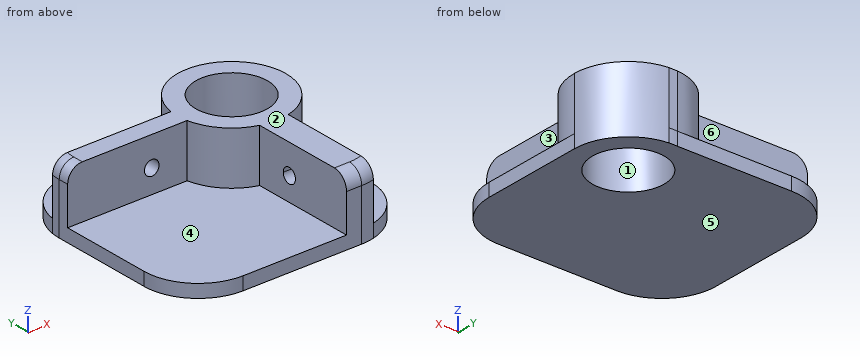
from build123d import *

# Parameters (mm, degrees)
F0_R     = 13.35
F1_DEPTH = 4.5
F2_DEPTH = 18
F5_DEPTH = 63.468562
F6_DEPTH = 56.501
F7_R     = 5
F8_R     = 13.35
F8_R_2   = 12.25
F9_DEPTH = 22.5


with BuildPart() as f1:
    # F0 (on Top) → F1 (new body)
    with BuildSketch(Plane.XY):
        with BuildLine():
            ThreePointArc((6.94, -57.959298), (17.066915, -51.404166), (21, -40))
            Line((21, -40), (21, -5))
            ThreePointArc((21, -5), (17.066915, -16.404166), (6.94, -22.959298))
            Line((6.94, -22.959298), (6.94, -57.959298))
        make_face()
        with Locations((2.5, -5)):
            Circle(F0_R)
        with BuildLine():
            ThreePointArc((6.94, -22.959298), (17.066915, -16.404166), (21, -5))
            ThreePointArc((21, -5), (16.086734, 7.555902), (3.956684, 13.442561))
            Line((3.956684, 13.442561), (1.066985, 13.444416))
            ThreePointArc((1.066985, 13.444416), (-10.011528, 8.627607), (-15.755136, -2))
            ThreePointArc((-15.755136, -2), (-15.998257, -5.25395), (-15.665902, -8.5))
            ThreePointArc((-15.665902, -8.5), (-11.178256, -17.456136), (-2.68, -22.76))
            ThreePointArc((-2.68, -22.76), (2.116816, -23.496031), (6.94, -22.959298))
        make_face()
        with Locations((2.5, -5)):
            Circle(F0_R, mode=Mode.SUBTRACT)
        with BuildLine():
            ThreePointArc((2.5, -58.5), (4.736401, -58.364327), (6.94, -57.959298))
            Line((6.94, -57.959298), (6.94, -22.959298))
            ThreePointArc((6.94, -22.959298), (2.116816, -23.496031), (-2.68, -22.76))
            Line((-2.68, -22.76), (-2.68, -58.5))
            Line((-2.68, -58.5), (2.5, -58.5))
        make_face()
        with BuildLine():
            Line((1.066985, 13.444416), (3.956684, 13.442561))
            ThreePointArc((3.956684, 13.442561), (2.511871, 13.499996), (1.066985, 13.444416))
        make_face()
        with BuildLine():
            ThreePointArc((-15.755136, -2), (-10.011528, 8.627607), (1.066985, 13.444416))
            Line((1.066985, 13.444416), (-38.015691, 13.469493))
            ThreePointArc((-38.015691, 13.469493), (-49.985176, 9.085639), (-56.277659, -2))
            Line((-56.277659, -2), (-15.755136, -2))
        make_face()
        with BuildLine():
            Line((-2.68, -58.5), (-2.68, -22.76))
            ThreePointArc((-2.68, -22.76), (-11.178256, -17.456136), (-15.665902, -8.5))
            Line((-15.665902, -8.5), (-56.527562, -8.5))
            Line((-56.527562, -8.5), (-56.527562, -40))
            ThreePointArc((-56.527562, -40), (-51.109037, -53.081475), (-38.027562, -58.5))
            Line((-38.027562, -58.5), (-2.68, -58.5))
        make_face()
        with BuildLine():
            ThreePointArc((-15.665902, -8.5), (-15.998257, -5.25395), (-15.755136, -2))
            Line((-15.755136, -2), (-56.277659, -2))
            ThreePointArc((-56.277659, -2), (-56.46498, -3.510108), (-56.527562, -5.030503))
            Line((-56.527562, -5.030503), (-56.527562, -8.5))
            Line((-56.527562, -8.5), (-15.665902, -8.5))
        make_face()
    extrude(amount=-F1_DEPTH)

    # F0 (on Top) → F2 (join)
    with BuildSketch(Plane.XY):
        with BuildLine():
            ThreePointArc((2.5, -58.5), (4.736401, -58.364327), (6.94, -57.959298))
            Line((6.94, -57.959298), (6.94, -22.959298))
            ThreePointArc((6.94, -22.959298), (2.116816, -23.496031), (-2.68, -22.76))
            Line((-2.68, -22.76), (-2.68, -58.5))
            Line((-2.68, -58.5), (2.5, -58.5))
        make_face()
        with BuildLine():
            ThreePointArc((6.94, -22.959298), (17.066915, -16.404166), (21, -5))
            ThreePointArc((21, -5), (16.086734, 7.555902), (3.956684, 13.442561))
            Line((3.956684, 13.442561), (1.066985, 13.444416))
            ThreePointArc((1.066985, 13.444416), (-10.011528, 8.627607), (-15.755136, -2))
            ThreePointArc((-15.755136, -2), (-15.998257, -5.25395), (-15.665902, -8.5))
            ThreePointArc((-15.665902, -8.5), (-11.178256, -17.456136), (-2.68, -22.76))
            ThreePointArc((-2.68, -22.76), (2.116816, -23.496031), (6.94, -22.959298))
        make_face()
        with Locations((2.5, -5)):
            Circle(F0_R, mode=Mode.SUBTRACT)
        with BuildLine():
            ThreePointArc((-15.665902, -8.5), (-15.998257, -5.25395), (-15.755136, -2))
            Line((-15.755136, -2), (-56.277659, -2))
            ThreePointArc((-56.277659, -2), (-56.46498, -3.510108), (-56.527562, -5.030503))
            Line((-56.527562, -5.030503), (-56.527562, -8.5))
            Line((-56.527562, -8.5), (-15.665902, -8.5))
        make_face()
    extrude(amount=F2_DEPTH)

    # F3 (on face) → F5 (cut, through all)
    with BuildSketch(Plane.YZ.offset(6.94)):
        with BuildLine():
            ThreePointArc((-32.459298, 8), (-33.191531, 9.767767), (-34.959298, 10.5))
            ThreePointArc((-34.959298, 10.5), (-36.727065, 6.232233), (-32.459298, 8))
        make_face()
    extrude(amount=-F5_DEPTH, mode=Mode.SUBTRACT)

    # F4 (on face) → F6 (cut, through all)
    with BuildSketch(Plane(origin=(0, -2, 0), x_dir=(-1, 0, 0), z_dir=(0, 1, 0))):
        with BuildLine():
            ThreePointArc((30.255136, 8), (29.522903, 9.767767), (27.755136, 10.5))
            ThreePointArc((27.755136, 10.5), (25.987369, 6.232233), (30.255136, 8))
        make_face()
    extrude(amount=-F6_DEPTH, mode=Mode.SUBTRACT)

    # F7
    f7_edges = [f1.edges().sort_by_distance(p)[0] for p in [
        (-56.527562, -6.765252, 18),
        (-0.09, -58.5, 18),
        (4.736401, -58.364327, 18),
    ]]
    fillet(f7_edges, radius=F7_R)

    # F8 (on face) → F9 (join, through all)
    with BuildSketch(Plane.XY.offset(18)):
        with Locations((2.5, -5)):
            Circle(F8_R)
        with Locations((2.5, -5)):
            Circle(F8_R_2, mode=Mode.SUBTRACT)
    extrude(amount=-F9_DEPTH)


solid = f1.part
The model under review builds one solid part; all positions refer to its coordinate system, in mm. Face numbers are marked on the shaded views. A direction names the side the tool comes from. Round coordinates to 2 decimals unless told otherwise and drop trailing zeros. Loops run counter-clockwise (first coordinate to the right, second up) from the corner with the lowest first, then second, coordinate; pieces in that order, holes last. Notation, with made-up numbers: M 49.5,45 L 76.5,45 A14 cw 76.5,51 Z; hole C 31,38 d11. An arc over 180 degrees is marked long. Answer as CSV lines item,"result". Start each with the question number.
Item 1: Wall thickness on line 1 (Y direction, x = 2.5, z = 1.75); line 2 (X direction, y = -6.75, z = 8); line 3 (Z direction, x = -28, y = -6): over which ranges is each line inside the solid? List them lowest first. Write a range as [from, to].
Item 2: Consider section C-C (y = -38.5). Write out the cut boundary in (x, z), then the cut area to 3 significant figures.
Item 3: Consider section A-A (z = 3.5). Write out the cut boundary in (x, y), then the cut area to 3 significant figures.
Item 4: For the marked faces 4, 5 and 6, list the 3-axis set-ups (+Z, -Z, +X, -X, +Y, -Y) from which the entire face can be reached by the end or side of a thin tool; tool diameter is ignored.
Item 5: Consider section D-D (x = -46.5). Write out the cut boundary in (y, z), then the cut area to 3 significant figures.
Item 6: Insertion check: P1, Ø9, axis at y = -48.5, z = 6.5, coming from the +X side; P2, Ø5.5, axis at y = -35.5, z = 8.5, coming from the -X side; P3, Ø5, axis at y = 3, z = 1.5, coming from the -X side. Each pin has a flat end and moves straight along its axis. Give the tip position at first contact, or say it passes through.
Item 7: Mouldability with a two-part tool opening along X and no side actions: class the marked faces 1, 2 and 3 as released by +X, released by -X, zero draft, split by the parting line, or undercut.
Item 8: Consider section B-B (x = -26.5). Write out the cut boundary in (y, z).
Answer:
1,line 1,"y = [-58.5, -17.25], [7.25, 13.44]"
1,line 2,"x = [-56.53, -30.26], [-25.26, -9.62], [14.62, 20.92]"
1,line 3,"z = [-4.5, 5.51], [10.49, 18]"
2,outline,"M -56.53,-4.5 L 21,-4.5 L 21,0 L 6.94,0 L 6.94,18 L -2.68,18 L -2.68,0 L -56.53,0 Z"
2,area,"522 mm^2"
3,outline,"M -56.53,-8.5 L -15.67,-8.5 A18.5 ccw -2.68,-22.76 L -2.68,-58.5 L 2.5,-58.5 A18.5 ccw 6.94,-57.96 L 6.94,-22.96 A18.5 ccw 21,-5 A18.5 ccw 3.96,13.44 L 1.07,13.44 A18.5 ccw -15.76,-2 L -56.28,-2 A18.5 ccw -56.53,-5.03 Z; hole C 2.5,-5 d24.5"
3,area,"1,210 mm^2"
4,face 4,"+Z, -X, -Y"
4,face 5,"-Z, +X, -X, +Y, -Y"
4,face 6,"+Z, -X, +Y"
5,outline,"M -56.45,-4.5 L 11.42,-4.5 L 11.42,0 L -2,0 L -2,18 L -8.5,18 L -8.5,0 L -56.45,0 Z"
5,area,"422 mm^2"
6,P1,"stops at x = 6.94"
6,P2,"stops at x = -2.68"
6,P3,"stops at x = -55.52"
7,face 1,"undercut"
7,face 2,"zero draft"
7,face 3,"released by +X"
8,outline,"M -58.5,-4.5 L 13.46,-4.5 L 13.46,0 L -2,0 L -2,5.84 L -8.5,5.84 L -8.5,0 L -58.5,0 Z; M -8.5,10.16 L -2,10.16 L -2,18 L -8.5,18 Z"
